Build history of the part. All positions in model axes, mm. Face numbers are marked on the shaded views. A direction names the side the tool comes from. Give positions to 0.01 mm unless a question says otherwise; leave off trailing zeros. Loops run counter-clockwise (first coordinate to the right, second up) from the corner with the lowest first, then second, coordinate; pieces in that order, holes last. Notation, with made-up numbers: M -11.75,62.25 L 6.25,62.25 A11 cw 6.25,74.25 Z; hole C -6,61 d5. An arc over 180 degrees is marked long. Answer in a Markdown table with one row per item. Add a question column.
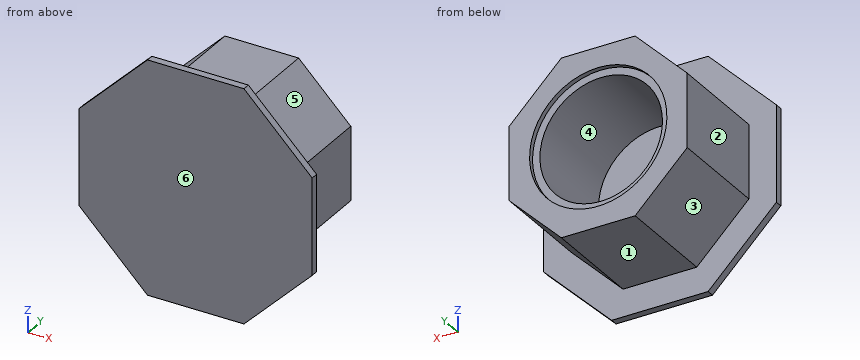
```python
from build123d import *

# Parameters (mm, degrees)
BOSS_EXTRUDE7_DEPTH = 6
SKETCH1_R           = 50
BOSS_EXTRUDE8_DEPTH = 84
CUT_EXTRUDE1_START  = -4
SKETCH4_R           = 56
SKETCH4_R_2         = 50
CUT_EXTRUDE1_DEPTH  = 4


with BuildPart() as part:
    # Sketch2 → Boss-Extrude7 (new body)
    with BuildSketch(Plane(origin=(0, 0, 0), x_dir=(1, 0, 0), z_dir=(0, 1, 0))):
        Polygon((39.35, -94.999303679), (94.999303679, -39.35), (94.999303679, 39.35), (39.35, 94.999303679), (-39.35, 94.999303679), (-94.999303679, 39.35), (-94.999303679, -39.35), (-39.35, -94.999303679), align=None)
    extrude(amount=-BOSS_EXTRUDE7_DEPTH)

    # Sketch1 → Boss-Extrude8 (add)
    with BuildSketch(Plane(origin=(0, 0, 0), x_dir=(1, 0, 0), z_dir=(0, 1, 0))):
        Polygon((-72.59, -30.067762493), (-30.067762493, -72.59), (30.067762493, -72.59), (72.59, -30.067762493), (72.59, 30.067762493), (30.067762493, 72.59), (-30.067762493, 72.59), (-72.59, 30.067762493), align=None)
        with Locations(Location((0, 0, 0), (0, 0, 90))):
            Circle(SKETCH1_R, mode=Mode.SUBTRACT)
    extrude(amount=BOSS_EXTRUDE8_DEPTH)

    # Sketch4 → Cut-Extrude1 (cut)
    with BuildSketch(Plane(origin=(0, 84, 0), x_dir=(1, 0, 0), z_dir=(0, 1, 0)).offset(CUT_EXTRUDE1_START)):
        with Locations(Location((0, 0, 0), (0, 0, 270))):
            Circle(SKETCH4_R)
        with Locations(Location((0, 0, 0), (0, 0, 90))):
            Circle(SKETCH4_R_2, mode=Mode.SUBTRACT)
    extrude(amount=CUT_EXTRUDE1_DEPTH, mode=Mode.SUBTRACT)


solid = part.part
```
(1) Slice it at D-D, the plane z = -64. Give the cut face in (x, y).
(2) Pull direction X, two halves, no side cores. Call the marked faces 4, 5 and 6: +X half, -X half, draft (parallel to the pull), parting line (faces both ways), or undercut.
(3) Slice it at B-B, the plane z = 0. Give the cut face in (x, y), then the cut area to 3 significant figures.
(4) Tool access for the marked faces 1, 2 and 3: list every direction of +Z, -Z, +X, -X, +Y, -Y with a clear straight run to the whole face (end or side of a thin tool).
(5) Slice it at C-C, the plane x = 0. Give the cut face in (y, z).
(6) Pin check, flat tips, straight feed: pin 1 (4 mm diameter, centred on x = -16.5, y = 30, fed in from -Z); pin 2 (12 mm diameter, centred on y = 20, z = -1, fed in from -X); pin 3 (8 mm diameter, centred on y = 6.5, z = -54, fed in from +X). Stop position of each tip, or through.
(7) Slice it at A-A, the plane y = 52. Give the cut face in (x, z).
(8) Wall check: line 1 (X direction, y = 25, z = 0); line 2 (X direction, y = 82, z = 0); line 3 (Y direction, x = 20, z = 79). Give the ranges that are in metal, low to high.
Solution:
| question | item | result |
|---|---|---|
| 1 | outline | M -70.35,-6 L 70.35,-6 L 70.35,0 L 38.66,0 L 38.66,84 L -38.66,84 L -38.66,0 L -70.35,0 Z |
| 2 | face 4 | undercut |
| 2 | face 5 | +X half |
| 2 | face 6 | draft |
| 3 | outline | M -95,-6 L 95,-6 L 95,0 L 72.59,0 L 72.59,84 L 56,84 L 56,80 L 50,80 L 50,0 L -50,0 L -50,80 L -56,80 L -56,84 L -72.59,84 L -72.59,0 L -95,0 Z |
| 3 | area | 4,890 mm^2 |
| 4 | face 1 | -Z, +X, -X, +Y |
| 4 | face 2 | +Z, -Z, -X, +Y |
| 4 | face 3 | -Z, -X, +Y |
| 5 | outline | M -6,-95 L 0,-95 L 0,-72.59 L 84,-72.59 L 84,-56 L 80,-56 L 80,-50 L 0,-50 L 0,50 L 80,50 L 80,56 L 84,56 L 84,72.59 L 0,72.59 L 0,95 L -6,95 Z |
| 6 | pin 1 | z = -72.59 |
| 6 | pin 2 | x = -72.59 |
| 6 | pin 3 | x = 52.66 |
| 7 | outline | M -72.59,-30.07 L -30.07,-72.59 L 30.07,-72.59 L 72.59,-30.07 L 72.59,30.07 L 30.07,72.59 L -30.07,72.59 L -72.59,30.07 Z; hole C 0,0 d100 |
| 8 | line 1 | -72.59 to -50, 50 to 72.59 |
| 8 | line 2 | -72.59 to -56, 56 to 72.59 |
| 8 | line 3 | -6 to 0 |
